Drawing for the job (mm, zero at the part's lowest x, y, z). A direction names the side the tool comes from. Round coordinates to 2 decimals unless told otherwise and drop trailing zeros. Order: outer loops, then holes, each group sorted by start corner. A loop starts at its lowest first (then second) coordinate and runs counter-clockwise, first axis right, second up. Notation, with made-up numbers: (-24.5, 74) - (6.5, 74) arc R29 cw to (6.5, 102) - close; hole circle Ø8 at (34.5, 40). An arc over 180 degrees is marked (long way). Put each result on its own line as item: value. Start each with the question number.
Item 1: Pin check, flat tips, straight feed: pin 1 Ø12.5 at (y, z) = (78, 83) entering from -X; pin 2 Ø2 at (x, z) = (183, 82.5) entering from -Y; pin 3 Ø12.5 at (x, z) = (80, 8) entering from -Y. Stop position of each tip, or through.
Item 2: Probe probe 1 along X at (y, z) = (7.5, 6.5); probe 2 along Z at (x, y) = (152, 44.5); probe 3 along Y at (x, z) = (131.5, 47). List the from-to ranges inside material, lowest first.
Item 3: Mould opens along X. For the marked faces 1, 2, 3 and 4 say: pulls with the +X half, pulls with the -X half, needs draft (parallel to the pull), parting line crosses it, or undercut.
Item 4: Saw through at B-B on y = 10.5. List the corners of the cut face in (x, z).
Item 5: Saw through at D-D on z = 15. List the corners of the cut face in (x, y).
Item 6: Which spindle directions (+Z, -Z, +X, -X, +Y, -Y) get a long thin tool onto all of the face, cutting with end or side? Do the marked faces 5, 6, 7, 8 and 9. Say none if no direction does.
Item 7: Saw through at C-C on y = 75.5. List the corners of the cut face in (x, z), plus the area to 3 significant figures.
Item 8: Saw through at A-A on z = 95. List the corners of the cut face in (x, y).
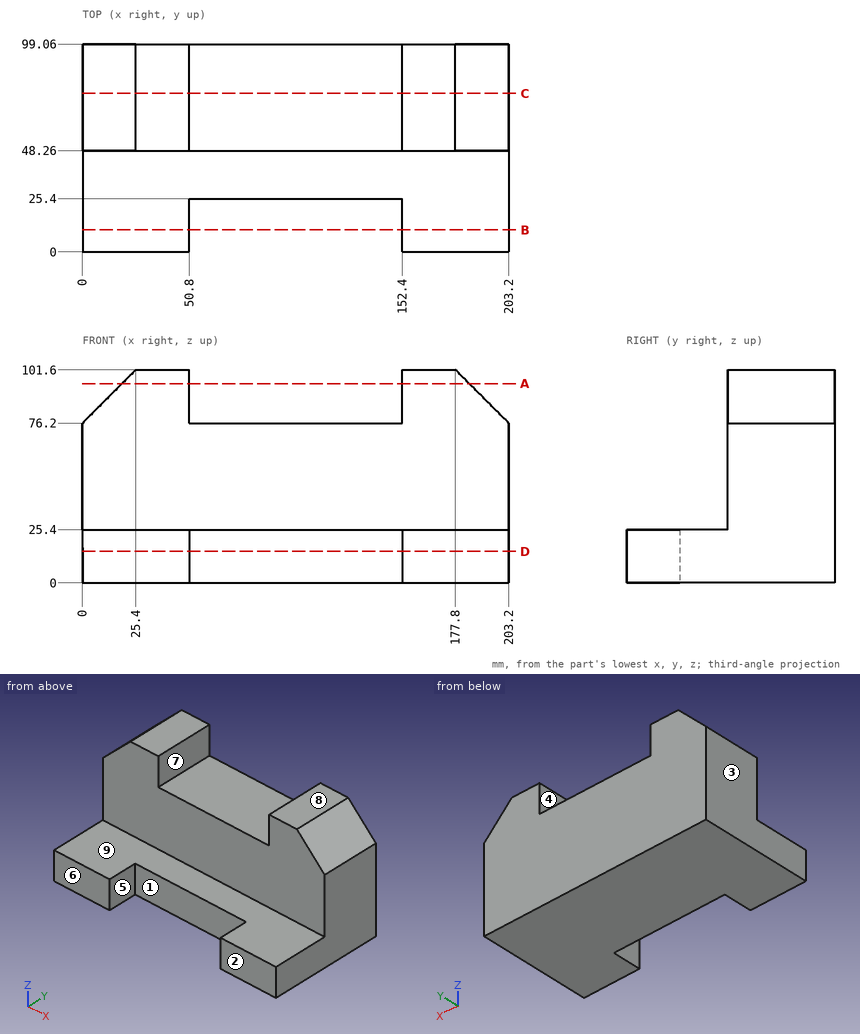
Results found:
1. pin 1: stops at x = 0.55
1. pin 2: stops at y = 48.26
1. pin 3: stops at y = 25.4
2. probe 1: x = 0 to 50.8, 152.4 to 203.2
2. probe 2: z = 0 to 25.4
2. probe 3: y = 48.26 to 99.06
3. face 1: undercut
3. face 2: needs draft
3. face 3: pulls with the -X half
3. face 4: undercut
4. outline: (0, 0) - (50.8, 0) - (50.8, 25.4) - (0, 25.4) - close; (152.4, 0) - (203.2, 0) - (203.2, 25.4) - (152.4, 25.4) - close
5. outline: (0, 0) - (50.8, 0) - (50.8, 25.4) - (152.4, 25.4) - (152.4, 0) - (203.2, 0) - (203.2, 99.06) - (0, 99.06) - close
6. face 5: +Z, -Z, -Y
6. face 6: +Z, -Z, +X, -X, -Y
6. face 7: +Z, +Y, -Y
6. face 8: +Z, +X, -X, +Y, -Y
6. face 9: +Z, +X, -X, -Y
7. outline: (0, 0) - (203.2, 0) - (203.2, 76.2) - (177.8, 101.6) - (152.4, 101.6) - (152.4, 76.2) - (50.8, 76.2) - (50.8, 101.6) - (25.4, 101.6) - (0, 76.2) - close
7. area: 17,400 mm²
8. outline: (18.8, 48.26) - (50.8, 48.26) - (50.8, 99.06) - (18.8, 99.06) - close; (152.4, 48.26) - (184.4, 48.26) - (184.4, 99.06) - (152.4, 99.06) - close
